CAD build for the part. Positions are in the model's coordinates, mm. A direction names the side the tool comes from. Coordinates: 2 decimals unless noted, no trailing zeros. Loops run counter-clockwise (first coordinate to the right, second up) from the corner with the lowest first, then second, coordinate; pieces in that order, holes last. Notation, with made-up numbers: (6, 78.25) -> (12, 78.25) arc R14 cw to (12, 88.25) -> close; hole circle Ø10 at (-31, 50.5). An arc over 180 degrees is marked (long way). Write each question's results on one line, items separated by ' | '.
from build123d import *

# Parameters (mm, degrees)
BOSS_EXTRUDE1_DEPTH     = 28.575
SKETCH2_W               = 1.00076
SKETCH2_H               = 1.5875
CUT_EXTRUDE2_DEPTH      = 41.5003
CUT_EXTRUDE2_DEPTH_BACK = 41.5003
SKETCH3_W               = 68.3006
SKETCH3_H               = 3.9878
BOSS_EXTRUDE2_DEPTH     = 21.0058
SKETCH4_W               = 56.4896
SKETCH4_H               = 29.0068
BOSS_EXTRUDE3_DEPTH     = 5.9944
SKETCH5_W               = 5.0038
SKETCH5_H               = 15.07744
CUT_EXTRUDE3_DEPTH      = 5.9944


with BuildPart() as part:
    # Sketch1 → Boss-Extrude1 (new body)
    with BuildSketch(Plane(origin=(0, 0, 0), x_dir=(1, 0, 0), z_dir=(0, 1, 0))):
        Polygon((-40.5003, 0), (40.5003, 0), (34.1503, -6.35), (-34.1503, -6.35), align=None)
    extrude(amount=BOSS_EXTRUDE1_DEPTH)

    # Sketch2 → Cut-Extrude2 (cut, two sides)
    with BuildSketch(Plane(origin=(0, 0, 0), x_dir=(0, 0, -1), z_dir=(1, 0, 0))) as cut_extrude2_sk:
        with Locations((-0.50038, 0.79375)):
            Rectangle(SKETCH2_W, SKETCH2_H)
    extrude(amount=CUT_EXTRUDE2_DEPTH, mode=Mode.SUBTRACT)
    extrude(cut_extrude2_sk.sketch, amount=-CUT_EXTRUDE2_DEPTH_BACK, mode=Mode.SUBTRACT)

    # Sketch3 → Boss-Extrude2 (add)
    with BuildSketch(Plane.XY.offset(6.35)):
        with Locations((0, 19.5707)):
            Rectangle(SKETCH3_W, SKETCH3_H)
    extrude(amount=BOSS_EXTRUDE2_DEPTH)

    # Sketch4 → Boss-Extrude3 (add)
    with BuildSketch(Plane.XY.offset(6.35)):
        with Locations((0, 3.0734)):
            Rectangle(SKETCH4_W, SKETCH4_H)
    extrude(amount=BOSS_EXTRUDE3_DEPTH)

    # Sketch5 → Cut-Extrude3 (cut)
    with BuildSketch(Plane.XY.offset(12.3444)):
        with Locations((-17.7419, 10.03808)):
            Rectangle(SKETCH5_W, SKETCH5_H)
        with Locations((17.2593, 10.03808)):
            Rectangle(SKETCH5_W, SKETCH5_H)
    extrude(amount=-CUT_EXTRUDE3_DEPTH, mode=Mode.SUBTRACT)


solid = part.part
1) Two-plate mould, pull along X, no slides. Class faces 1 (the flat face through (0, 25, 6.35)), 2 (the flat face through (-18, 2.499, 9)), 3 (the flat face through (-37.3, 14.1, 3.2)), 4 (the flat face through (17, 2.499, 9)): pulls with the +X half, pulls with the -X half, needs draft (parallel to the pull), parting line crosses it, or undercut.
Outcome:
face 1: needs draft | face 2: undercut | face 3: pulls with the -X half | face 4: undercut
2) Slice it at B-B (y = 15). Write the cut outline in (x, z), then the cut area to 3 significant figures.
Outcome:
outline: (-40.5, 0) -> (40.5, 0) -> (34.15, 6.35) -> (28.24, 6.35) -> (28.24, 12.34) -> (19.76, 12.34) -> (19.76, 6.35) -> (14.76, 6.35) -> (14.76, 12.34) -> (-15.24, 12.34) -> (-15.24, 6.35) -> (-20.24, 6.35) -> (-20.24, 12.34) -> (-28.24, 12.34) -> (-28.24, 6.35) -> (-34.15, 6.35) -> close | area: 753 mm^2
3) Which spindle directions (+Z, -Z, +X, -X, +Y, -Y) get a long thin tool onto all of the face, cutting with end or side? Do faces 5 (the flat face through (1, 0, 4)), 6 (the flat face through (31, 9, 6.35)), 7 (the flat face through (0, 21.565, 17)), 8 (the flat face through (-20.244, 10, 9)), 9 (the flat face through (-28.245, 3, 9)). Say none if no direction does.
Outcome:
face 5: -Z, +X, -X, -Y | face 6: +Z, +X, -Y | face 7: +Z, +X, -X, +Y | face 8: +Z | face 9: +Z, -X, -Y
4) Slice it at D-D (y = -3). Write the cut outline in (x, z), then the cut area to 3 significant figures.
Outcome:
outline: (-28.24, 6.35) -> (28.24, 6.35) -> (28.24, 12.34) -> (-28.24, 12.34) -> close | area: 339 mm^2
5) Pin check, flat tips, straight feed: pin 1 (6.5 mm diameter, centred on y = 4.5, z = 9, fed in from +X); pin 2 (5 mm diameter, centred on y = 9.5, z = 8.5, fed in from -X); pin 3 (1.5 mm diameter, centred on y = 23.5, z = 10, fed in from +X); pin 4 (8 mm diameter, centred on x = -24, y = 1.5, fed in from +Z). Stop position of each tip, or through.
Outcome:
pin 1: stops at x = 34.75 | pin 2: stops at x = -34.5 | pin 3: passes through | pin 4: stops at z = 12.34
6) Drill centre lines: L1, parallel to X at y = 16, z = 11.5; L2, parallel to Z at x = -8.5, y = 9; L3, parallel to Y at x = 20, z = 13. Where is each one in solid material? Low to high. Write a range as from..to.
Outcome:
L1: x = -28.24..-20.24, -15.24..14.76, 19.76..28.24 | L2: z = 0..12.34 | L3: y = 17.58..21.56
7) Slice it at C-C (z = 19.75). Write the cut outline in (x, y).
Outcome:
outline: (-34.15, 17.58) -> (34.15, 17.58) -> (34.15, 21.56) -> (-34.15, 21.56) -> close
